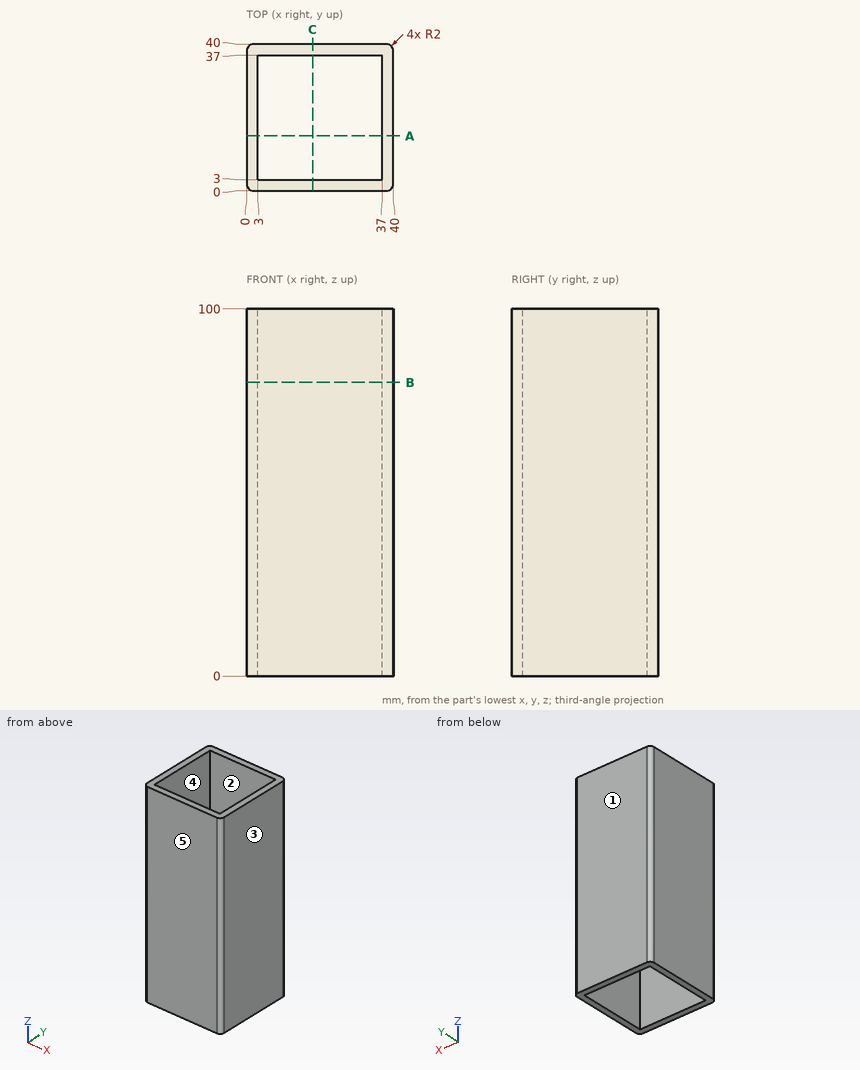
Answer from the drawing. Dimensions are ordinates in mm from the lowest x, y and z of the part. A direction names the side the tool comes from. Give positions to 0.01 mm unless a question says otherwise; leave off trailing zeros. Order: outer loops, then holes, each group sorted by start corner. A loop starts at its lowest first (then second) coordinate and runs counter-clockwise, first axis right, second up. Notation, with made-up numbers: (23, 54) - (27, 54) arc R19 cw to (27, 91) - close; hole circle Ø6 at (19, -18). An arc over 180 degrees is marked (long way). Use one line per item in the form item = value.
1) For the marked faces 1 and 2, determine the directions among +Z, -Z, +X, -X, +Y, -Y from which every point of the face is accessible in a straight line to the end or side of a thin tool.
Verdict:
face_1 = +Z, -Z, +X, -X, +Y
face_2 = +Z, -Z
2) Find section B-B on z = 80. Determine the outline of the cut face in (x, y), and give its area (3 significant figures).
Verdict:
outline = (0, 2) arc R2 ccw to (2, 0) - (38, 0) arc R2 ccw to (40, 2) - (40, 38) arc R2 ccw to (38, 40) - (2, 40) arc R2 ccw to (0, 38) - close; hole (3, 3) - (37, 3) - (37, 37) - (3, 37) - close
area = 441 mm^2
3) Find section A-A on y = 15. Determine the outline of the cut face in (x, z), and give its area (3 significant figures).
Verdict:
outline = (0, 0) - (3, 0) - (3, 100) - (0, 100) - close; (37, 0) - (40, 0) - (40, 100) - (37, 100) - close
area = 600 mm^2
4) The mould has two halves that part along X. Classify the marked faces 3, 4 and 5: released by +X, released by -X, zero draft, split by the parting line, or undercut.
Verdict:
face_3 = released by +X
face_4 = undercut
face_5 = zero draft
5) Consider probe 1 along Y at (x, z) = (11.5, 46); probe 2 along Y at (x, z) = (38.5, 68.5). Determine where each line is inside the solid, lowest interval first. Write a range as [from, to].
Verdict:
probe_1 = [0, 3], [37, 40]
probe_2 = [0.06, 39.94]
